Could you check a few things on this model? Use its own coordinates, in mm. A direction names the side the tool comes from. Round coordinates to 2 decimals unless told otherwise and drop trailing zeros. Write each loop counter-clockwise with the first axis right and the second up, starting at its lowest first coordinate (ties: lowest second). Pieces come first, ordered by that corner, then holes. Notation, with made-up numbers: (-17, 47.25) -> (33, 47.25) arc R26 cw to (33, 74.25) -> close; hole circle Ø4 at (78, -21). An arc over 180 degrees is marked (long way). Answer in a Markdown table with one row per item.
from build123d import *

# Parameters (mm, degrees)
SKETCH1_R           = 6.35
BOSS_EXTRUDE1_DEPTH = 2.54
FILLET2_R           = 1.27
SKETCH2_R           = 3.96875
BOSS_EXTRUDE3_DEPTH = 17.78


with BuildPart() as part:
    # Sketch1 → Boss-Extrude1 (new body)
    with BuildSketch(Plane(origin=(0, 0, 0), x_dir=(1, 0, 0), z_dir=(0, 1, 0))):
        Circle(SKETCH1_R)
    extrude(amount=BOSS_EXTRUDE1_DEPTH)

    # Fillet2
    fillet2_edges = [part.edges().sort_by_distance(p)[0] for p in [
        (-6.35, 0, 0),
    ]]
    fillet(fillet2_edges, radius=FILLET2_R)

    # Sketch2 → Boss-Extrude3 (add)
    with BuildSketch(Plane(origin=(0, 2.54, 0), x_dir=(1, 0, 0), z_dir=(0, 1, 0))):
        Circle(SKETCH2_R)
    extrude(amount=BOSS_EXTRUDE3_DEPTH)


solid = part.part
1) Imagine slicing it at C-C, the plane y = 8.75. Please give me the cut outline in (x, z).
Findings:
| item | result |
|---|---|
| outline | circle Ø7.94 at (0, 0) |
2) For faces 1 (the face through (3, 2.54, -3)), 2 (the face through (0, 0, 0)), which set-ups out of +Z, -Z, +X, -X, +Y, -Y let a thin tool reach every point of the face, with its end or its side?
Findings:
| item | result |
|---|---|
| face 1 | +Y |
| face 2 | +Z, -Z, +X, -X, -Y |
3) Imagine slicing it at A-A, the plane x = 0. Please give me the cut outline in (y, z), plus the area to 3 significant figures.
Findings:
| item | result |
|---|---|
| outline | (0, -5.08) arc R1.27 ccw to (1.27, -6.35) -> (2.54, -6.35) -> (2.54, -3.97) -> (20.32, -3.97) -> (20.32, 3.97) -> (2.54, 3.97) -> (2.54, 6.35) -> (1.27, 6.35) arc R1.27 ccw to (0, 5.08) -> close |
| area | 173 mm^2 |
4) For pin 1 (1.5 mm diameter, centred on y = 2, z = -4.5, fed in from -X); pin 2 (1 mm diameter, centred on x = -1, y = 12, fed in from -Z); pin 3 (1.5 mm diameter, centred on y = 9, z = 4, fed in from +X), each with a flat end and sliding along its axis, tell me the tip position at first contact or that it passes through.
Findings:
| item | result |
|---|---|
| pin 1 | stops at x = -5.12 |
| pin 2 | stops at z = -3.94 |
| pin 3 | stops at x = 2.28 |
5) Imagine slicing it at B-B, the plane z = 0. Please give me the cut outline in (x, y), plus the area to 3 significant figures.
Findings:
| item | result |
|---|---|
| outline | (-6.35, 1.27) arc R1.27 ccw to (-5.08, 0) -> (5.08, 0) arc R1.27 ccw to (6.35, 1.27) -> (6.35, 2.54) -> (3.97, 2.54) -> (3.97, 20.32) -> (-3.97, 20.32) -> (-3.97, 2.54) -> (-6.35, 2.54) -> close |
| area | 173 mm^2 |
6) Please list where these lines run through material, in increasing order: line 1 (X direction, y = 5.75, z = 1.75); line 2 (Y direction, x = 4.5, z = 3); line 3 (Z direction, x = -2.5, y = 5.5).
Findings:
| item | result |
|---|---|
| line 1 | x = -3.56 to 3.56 |
| line 2 | y = 0.04 to 2.54 |
| line 3 | z = -3.08 to 3.08 |
